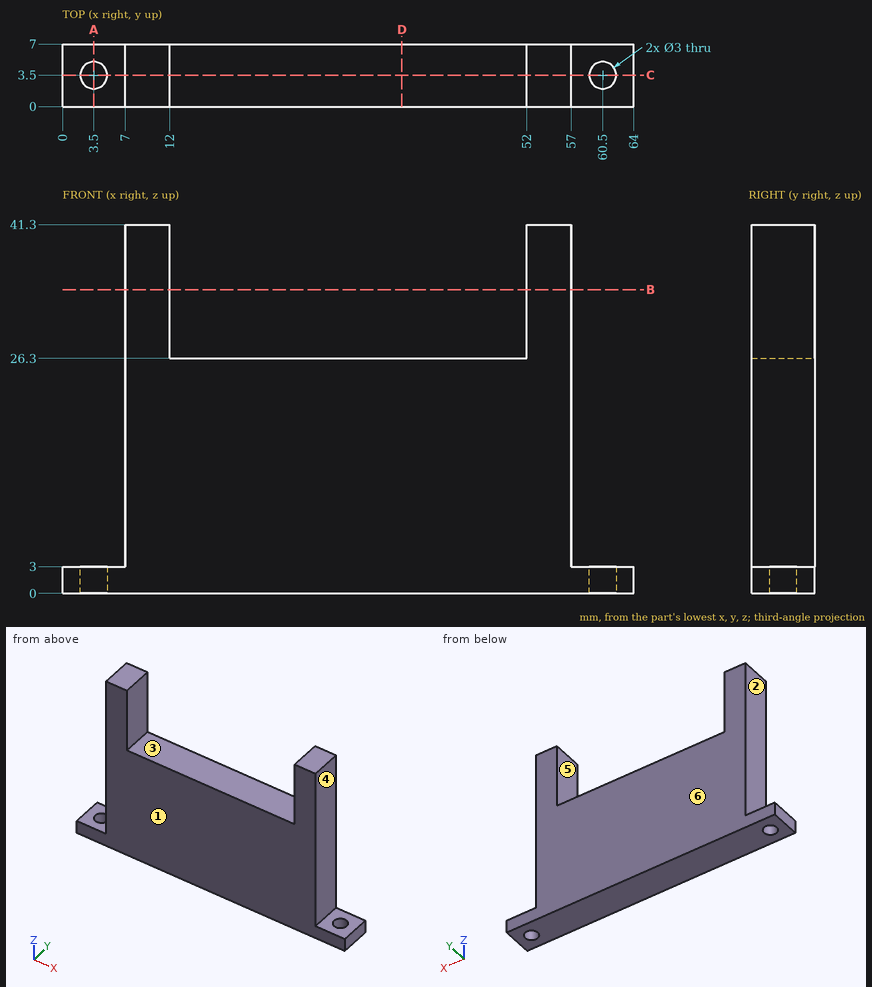
Design review of the part shown in the three views and the two pictorial views. Dimensions are in mm from the part's minimum x, y and z. A direction names the side the tool comes from. Round coordinates to 2 decimals unless told otherwise and drop trailing zeros. Write each loop counter-clockwise with the first axis right and the second up, starting at its lowest first coordinate (ties: lowest second). Pieces come first, ordered by that corner, then holes. Notation, with made-up numbers: (53, 5) - (59, 5) arc R21 ccw to (59, 22) - close; hole circle Ø5 at (64, 22). An arc over 180 degrees is marked (long way). Return JSON: item names as keys, results as strings. Group by question number.
Item 1: We need section A-A on x = 3.5. Write out the cut boundary in (y, z).
Item 2: The part is to be moulded in two halves that separate along X. For the marked faces 1, 2, 3 and 4, say which applies: pulls with the +X half, pulls with the -X half, needs draft (parallel to the pull), parting line crosses it, or undercut.
Item 3: For probe 1 along Y at (x, z) = (3.5, 1.1); probe 2 along X at (y, z) = (6.75, 25); probe 3 along Z at (x, y) = (46.5, 3.25), list the stretches that pass through material, from the lowest coordinate up. Write a range as [from, to].
Item 4: Machinability: for the marked faces 5 and 6, which of the approach directions +Z, -Z, +X, -X, +Y, -Y give a long, thin tool a straight path to every point of the face, cutting with its end or side? Answer none if there is none.
Item 5: We need section B-B on z = 34. Write out the cut boundary in (x, y), and give its area (3 significant figures).
Item 6: Insertion check: P1, Ø3, axis at y = 2.5, z = 32, coming from the -X side; P2, Ø2, axis at x = 32, y = 2, coming from the +Z side; P3, Ø3.5, axis at x = 60.5, y = 2, coming from the +Z side. Each pin has a flat end and moves straight along its axis. Give the tip position at first contact, or say it passes through.
Item 7: We need section D-D on x = 38. Write out the cut boundary in (y, z), and give its area (3 significant figures).
Item 8: We need section C-C on y = 3.5. Write out the cut boundary in (x, z).
Model answer:
{
 "1": {"outline": "(0, 0) - (2, 0) - (2, 3) - (0, 3) - close; (5, 0) - (7, 0) - (7, 3) - (5, 3) - close"},
 "2": {"face 1": "needs draft", "face 2": "pulls with the -X half", "face 3": "undercut", "face 4": "pulls with the +X half"},
 "3": {"probe 1": "y = [0, 2], [5, 7]", "probe 2": "x = [7, 57]", "probe 3": "z = [0, 26.3]"},
 "4": {"face 5": "+Z, +Y, -Y", "face 6": "+Z, -Z, +X, -X, +Y"},
 "5": {"outline": "(7, 0) - (12, 0) - (12, 7) - (7, 7) - close; (52, 0) - (57, 0) - (57, 7) - (52, 7) - close", "area": "70.0 mm²"},
 "6": {"P1": "stops at x = 7", "P2": "stops at z = 26.3", "P3": "stops at z = 3"},
 "7": {"outline": "(0, 0) - (7, 0) - (7, 26.3) - (0, 26.3) - close", "area": "184 mm²"},
 "8": {"outline": "(0, 0) - (2, 0) - (2, 3) - (0, 3) - close; (5, 0) - (59, 0) - (59, 3) - (57, 3) - (57, 41.3) - (52, 41.3) - (52, 26.3) - (12, 26.3) - (12, 41.3) - (7, 41.3) - (7, 3) - (5, 3) - close; (62, 0) - (64, 0) - (64, 3) - (62, 3) - close"}
}
